Geometry: final body of the model. Coordinates: model frame, mm. Face numbers are marked on the shaded views. Coordinates: 2 decimals unless noted, no trailing zeros. Loops run counter-clockwise (first coordinate to the right, second up) from the corner with the lowest first, then second, coordinate; pieces in that order, holes last. Notation, with made-up numbers: (22, 31) - (69, 31) arc R22 ccw to (69, 45) - close; hole circle Ø2 at (21.25, 11). An arc over 180 degrees is marked (long way). Answer in a Markdown table with one row per item.
Autodesk Inventor part; units mm, degrees
ref_plane "YZ Plane" through (0, 0, 0) normal (1, 0, 0) x (0, 1, 0)
ref_plane "XZ Plane" through (0, 0, 0) normal (0, 1, 0) x (-1, 0, 0)
ref_plane "XY Plane" through (0, 0, 0) normal (0, 0, 1) x (1, 0, 0)
sketch "スケッチ1" plane through (0, 0, 0) normal (1, 0, 0) x (0, 1, 0)
  line L0 (0, 0) -> (15, 0) construction
  line L1 (15, 0) -> (15, -40) construction
  line L2 (15, -40) -> (16, -40)
  line L3 (16, -40) -> (16, 10)
  line L4 (16, 10) -> (15, 10)
  line L5 (15, 10) -> (15, -40)
  line L6 (0, -50) -> (0, 20)
  dimension "d0" = 15
  dimension "d2" = 1
  dimension "d3" = 50
revolve "回転1" add sketch "スケッチ1" angle 180 about axis through (0, 0, -10) along (0, 0, 1)
sketch "スケッチ2" plane through (0, 15, 10) normal (1, 0, 0) x (0, 0, -1)
  line L0 (50, 1) -> (0, 1)
  line L1 (0, 1) -> (21, 1)
  line L2 (21, 1) -> (29, 1)
  line L3 (29, 1) -> (29, -6)
  line L4 (29, -6) -> (21, -6)
  line L5 (21, -6) -> (21, 1)
  line L6 (0, 1) -> (0, 0)
  point P0 (10, -15)
  point P1 (29, 1)
  dimension "d6" = 8
  dimension "d7" = 7
  dimension "d10" = 21
extrude "押し出し1" cut sketch "スケッチ2" against normal through all
properties part number "cover-pipe_L50" material "ステンレス鋼"
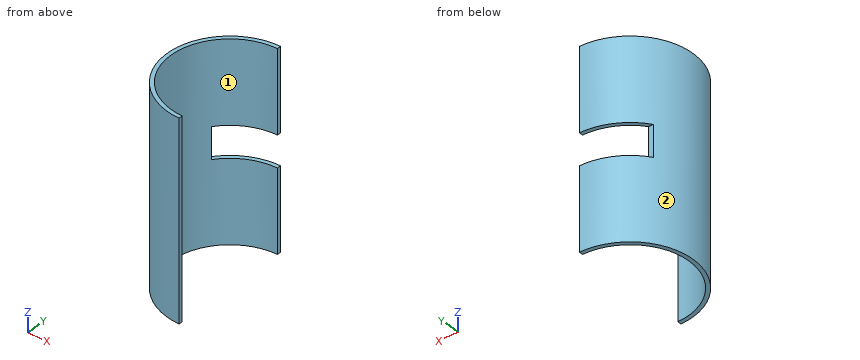
(1) First-contact query: pin 1 Ø2 at (x, z) = (-11.5, 4.5) entering from +Y; pin 2 Ø2 at (y, z) = (-5, -0.5) entering from +X; pin 3 Ø6 at (y, z) = (7.5, -4.5) entering from -X; pin 4 Ø2 at (x, y) = (-4, 14) entering from +Z. Flat tips, straight axial feed; report the tip coordinate or a pass-through.
Verdict:
| item | result |
|---|---|
| pin 1 | stops at y = 12.07 |
| pin 2 | stops at x = -13.75 |
| pin 3 | stops at x = -15.35 |
| pin 4 | stops at z = 10 |
(2) Pull-direction query (Y, two-part tool) for the marked faces 1 and 2; classes: pulls with the +Y half, pulls with the -Y half, needs draft (parallel to the pull), parting line crosses it, or undercut.
Verdict:
| item | result |
|---|---|
| face 1 | undercut |
| face 2 | parting line crosses it |
(3) Cut plane C-C on x = -6.5. Output: boundary loops of the cut face in (y, z).
Verdict:
| item | result |
|---|---|
| outline | (-14.62, -40) - (-13.52, -40) - (-13.52, 10) - (-14.62, 10) - close; (13.52, -40) - (14.62, -40) - (14.62, -19) - (13.52, -19) - close; (13.52, -11) - (14.62, -11) - (14.62, 10) - (13.52, 10) - close |
(4) Ray query, probe 1 along Z at (x, y) = (-7, 13.5); probe 2 along Y at (x, z) = (-1, 3.5); probe 3 along Y at (x, z) = (-4.25, -33.5). Return the intervals inside material, ascending.
Verdict:
| item | result |
|---|---|
| probe 1 | z = -40 to -19, -11 to 10 |
| probe 2 | y = -15.97 to -14.97, 14.97 to 15.97 |
| probe 3 | y = -15.43 to -14.39, 14.39 to 15.43 |
(5) Cut plane B-B on z = -1. Output: boundary loops of the cut face in (x, y).
Verdict:
| item | result |
|---|---|
| outline | (0, -16) - (0, -15) arc R15 cw to (0, 15) - (0, 16) arc R16 ccw to start |
(6) Cut plane A-A on x = -4.25. Output: boundary loops of the cut face in (y, z), then the cut area to 3 significant figures.
Verdict:
| item | result |
|---|---|
| outline | (-15.43, -40) - (-14.39, -40) - (-14.39, 10) - (-15.43, 10) - close; (14.39, -40) - (15.43, -40) - (15.43, -19) - (14.39, -19) - close; (14.39, -11) - (15.43, -11) - (15.43, 10) - (14.39, 10) - close |
| area | 95.7 mm² |
(7) Cut plane D-D on y = 0. Output: boundary loops of the cut face in (x, z).
Verdict:
| item | result |
|---|---|
| outline | (-16, -40) - (-15, -40) - (-15, 10) - (-16, 10) - close |
